from build123d import *

# Parameters (mm, degrees)
SKETCH1_W           = 50
SKETCH1_H           = 50
BOSS_EXTRUDE1_DEPTH = 29
SKETCH2_R           = 10
CUT_EXTRUDE1_DEPTH  = 40
SKETCH5_R           = 1.5
SKETCH5_R_2         = 4
CUT_EXTRUDE2_DEPTH  = 11
SKETCH6_R           = 20
CUT_EXTRUDE3_DEPTH  = 12
SKETCH7_R           = 18
CUT_EXTRUDE4_DEPTH  = 1


with BuildPart() as part:
    # Sketch1 → Boss-Extrude1 (new body, symmetric)
    with BuildSketch(Plane(origin=(0, 0, 0), x_dir=(1, 0, 0), z_dir=(0, 1, 0))):
        Rectangle(SKETCH1_W, SKETCH1_H)
    extrude(amount=BOSS_EXTRUDE1_DEPTH, both=True)

    # Sketch2 → Cut-Extrude1 (cut)
    with BuildSketch(Plane.ZY.offset(25)):
        Circle(SKETCH2_R)
    extrude(amount=-CUT_EXTRUDE1_DEPTH, mode=Mode.SUBTRACT)

    # Sketch5 → Cut-Extrude2 (cut, through all)
    with BuildSketch(Plane.ZY.offset(-15)):
        with Locations((0, 6.5)):
            Circle(SKETCH5_R)
        Circle(SKETCH5_R_2)
    extrude(amount=-CUT_EXTRUDE2_DEPTH, mode=Mode.SUBTRACT)

    # Sketch6 → Cut-Extrude3 (cut)
    with BuildSketch(Plane(origin=(0, 29, 0), x_dir=(1, 0, 0), z_dir=(0, 1, 0))):
        Circle(SKETCH6_R)
    cut_extrude3 = extrude(amount=-CUT_EXTRUDE3_DEPTH, mode=Mode.SUBTRACT)

    # Sketch7 → Cut-Extrude4 (cut)
    with BuildSketch(Plane(origin=(0, 17, 0), x_dir=(1, 0, 0), z_dir=(0, 1, 0))):
        Circle(SKETCH7_R)
    cut_extrude4 = extrude(amount=-CUT_EXTRUDE4_DEPTH, mode=Mode.SUBTRACT)

    # Mirror1: Cut-Extrude3, Cut-Extrude4 across plane
    add(cut_extrude3.mirror(Plane.ZX), mode=Mode.SUBTRACT)
    add(cut_extrude4.mirror(Plane.ZX), mode=Mode.SUBTRACT)


solid = part.part
CAD build for the part. Positions are in the model's coordinates, mm. A direction names the side the tool comes from. Coordinates: 2 decimals unless noted, no trailing zeros. Loops run counter-clockwise (first coordinate to the right, second up) from the corner with the lowest first, then second, coordinate; pieces in that order, holes last. Notation, with made-up numbers: (19.5, 29) - (74.5, 29) arc R23 ccw to (74.5, 42) - close; hole circle Ø5 at (9, 89). An arc over 180 degrees is marked (long way). Write item = value, one per line. Start each with the question number.
Q1. Cut at A-A, the plane y = 0. List the corners of the cut face in (x, z), then the cut area to 3 significant figures.
Q2. Drill centre lines: L1, parallel to Y at x = 19.25, z = 0; L2, parallel to Z at x = 0, y = -16.5; L3, parallel to Y at x = -4, z = 0. Where is each one in solid material? Low to high.
Q3. Cut at C-C, the plane z = 0. Give the number of separate pieces and of enclosed holes in the cut face, then the cut area to 3 significant figures.
Q4. Cut at B-B, the plane x = 0. List the corners of the cut face in (y, z).
Q5. Which spindle directions (+Z, -Z, +X, -X, +Y, -Y) get a long thin tool onto all of the face, cutting with end or side? Do faces 1 (the flat face through (0, -16, 0)), 2 (the flat face through (-18, 17, -3)), 3 (the flat face through (15, -4.3, -0.1)). Say none if no direction does.
Q6. Flat gauge pins, fed straight in: pin 1 Ø1.8 at (y, z) = (6.5, 0) entering from +X; pin 2 Ø12 at (x, z) = (3, 7.5) entering from -Y; pin 3 Ø10 at (y, z) = (-0.5, -3) entering from -X; pin 4 Ø24 at (x, z) = (0, 0) entering from +Y. Where does each tip first touch, or does it go through?
Q7. Pull direction Y, two halves, no side cores. Call faces 4 (the flat face through (-18, -17, -3)), 5 (the cylindrical face through (20, 5, 0)), 6 (the flat face through (0, 0, -25)): pulls with the +Y half, pulls with the -Y half, needs draft (parallel to the pull), parting line crosses it, or undercut.
Q8. Cut at D-D, the plane y = 21. List the corners of the cut face in (x, z), then the cut area to 3 significant figures.
Computed:
q1.outline = (-25, -25) - (25, -25) - (25, -4) - (15, -4) - (15, -10) - (-25, -10) - close; (-25, 10) - (15, 10) - (15, 4) - (25, 4) - (25, 25) - (-25, 25) - close
q1.area = 1,620 mm²
q2.L1 = -17 to -4, 4 to 5, 8 to 17
q2.L2 = -25 to -18, 18 to 25
q2.L3 = -16 to -10, 10 to 16
q3.separate_pieces = 3
q3.enclosed_holes = 0
q3.area = 958 mm²
q4.outline = (-29, -25) - (29, -25) - (29, -20) - (17, -20) - (17, -18) - (16, -18) - (16, 18) - (17, 18) - (17, 20) - (29, 20) - (29, 25) - (-29, 25) - (-29, 20) - (-17, 20) - (-17, 18) - (-16, 18) - (-16, -18) - (-17, -18) - (-17, -20) - (-29, -20) - close; hole circle Ø20 at (0, 0)
q5.face_1 = -Y
q5.face_2 = +Y
q5.face_3 = -X
q6.pin_1 = through
q6.pin_2 = -16
q6.pin_3 = 15
q6.pin_4 = 16
q7.face_4 = pulls with the -Y half
q7.face_5 = undercut
q7.face_6 = needs draft
q8.outline = (-25, -25) - (25, -25) - (25, 25) - (-25, 25) - close; hole circle Ø40 at (0, 0)
q8.area = 1,240 mm²
